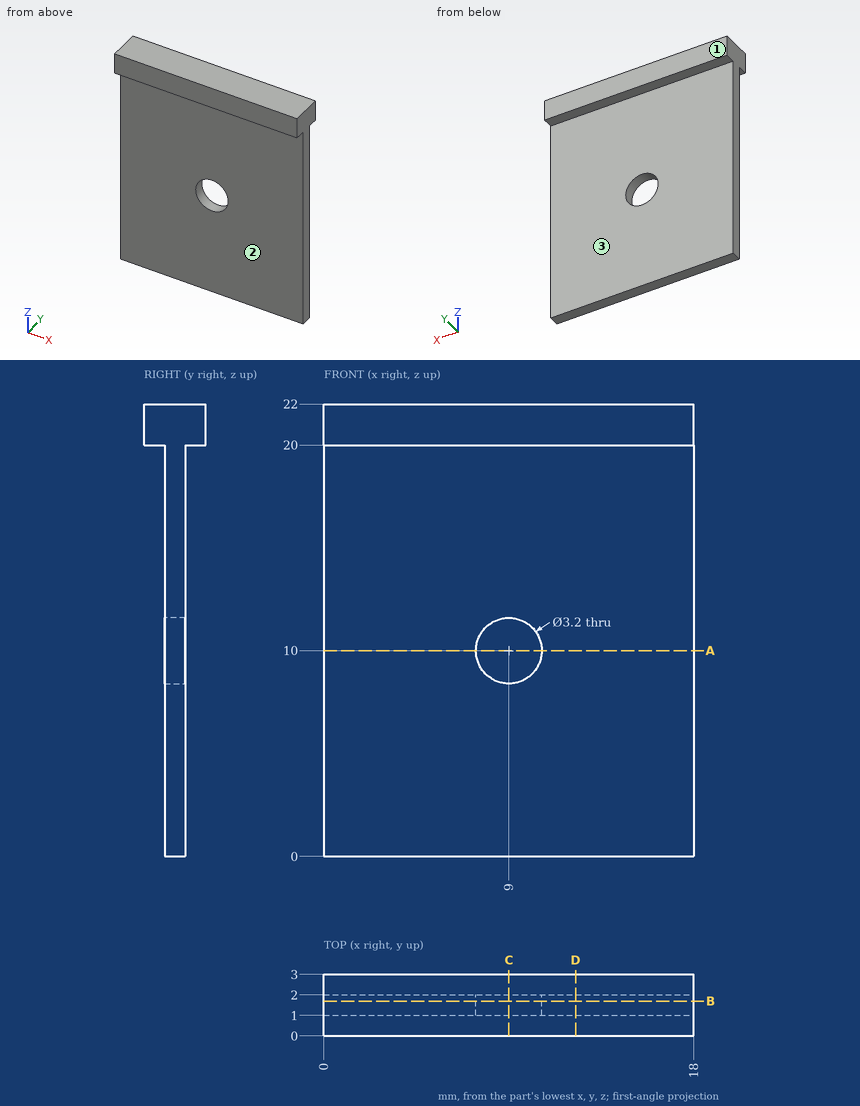
Can you work these out from the drawing? Everything is in mm from the part's minimum corner. A direction names the side the tool comes from. Coordinates: 2 decimals unless noted, no trailing zeros. Write each loop counter-clockwise with the first axis right and the second up, starting at its lowest first coordinate (ties: lowest second). Pieces come first, ordered by that corner, then holes. Notation, with made-up numbers: (-21, 29) - (-12, 29) arc R8 ccw to (-12, 38) - close; hole circle Ø4 at (71.25, -21.5). An arc over 180 degrees is marked (long way). Use a Markdown table: item, result.
Q1. Please list where these lines run through material, in increasing order: L1, parallel to X at y = 1.65, z = 10; L2, parallel to Y at x = 12.75, z = 14.5; L3, parallel to Z at x = 5.5, y = 0.95.
Geometry check:
| item | result |
|---|---|
| L1 | x = 0 to 7.4, 10.6 to 18 |
| L2 | y = 1 to 2 |
| L3 | z = 20 to 22 |
Q2. I'm going to push flat-ended pins straight in: pin 1 Ø0.5 at (x, y) = (10.5, 2.5) entering from -Z; pin 2 Ø6 at (x, z) = (13.5, 12.5) entering from +Y; pin 3 Ø10 at (x, z) = (11.5, 2.5) entering from -Y. Where does each tip first touch, or does it pass through?
Geometry check:
| item | result |
|---|---|
| pin 1 | stops at z = 20 |
| pin 2 | stops at y = 2 |
| pin 3 | stops at y = 1 |
Q3. Imagine slicing it at C-C (x = 9). List the corners of the cut face in (y, z) for me.
Geometry check:
| item | result |
|---|---|
| outline | (0, 20) - (1, 20) - (1, 11.6) - (2, 11.6) - (2, 20) - (3, 20) - (3, 22) - (0, 22) - close; (1, 0) - (2, 0) - (2, 8.4) - (1, 8.4) - close |
Q4. Imagine slicing it at A-A (z = 10). List the corners of the cut face in (x, y) for me.
Geometry check:
| item | result |
|---|---|
| outline | (0, 1) - (7.4, 1) - (7.4, 2) - (0, 2) - close; (10.6, 1) - (18, 1) - (18, 2) - (10.6, 2) - close |
Q5. Imagine slicing it at B-B (y = 1.7). List the corners of the cut face in (x, z) for me.
Geometry check:
| item | result |
|---|---|
| outline | (0, 0) - (18, 0) - (18, 22) - (0, 22) - close; hole circle Ø3.2 at (9, 10) |
Q6. Which directions (+Z, -Z, +X, -X, +Y, -Y) give clear straight access to the entire face, cutting with the end or side of a thin tool? Please do the marked faces 1, 2 and 3.
Geometry check:
| item | result |
|---|---|
| face 1 | +Z, -Z, +X, -X, +Y |
| face 2 | -Z, +X, -X, -Y |
| face 3 | -Z, +X, -X, +Y |
Q7. Imagine slicing it at D-D (x = 12.25). List the corners of the cut face in (y, z) for me, and give its area (3 significant figures).
Geometry check:
| item | result |
|---|---|
| outline | (0, 20) - (1, 20) - (1, 0) - (2, 0) - (2, 20) - (3, 20) - (3, 22) - (0, 22) - close |
| area | 26.0 mm2 |
